Here's the drawing with two shaded views (mm, measured from the low corner). I have some questions. Coordinates: 2 decimals unless noted, no trailing zeros. Order: outer loops, then holes, each group sorted by start corner. A loop starts at its lowest first (then second) coordinate and runs counter-clockwise, first axis right, second up. Notation, with made-up numbers: (37, 85.5) - (76, 85.5) arc R22 cw to (76, 104.5) - close; hole circle Ø11 at (43.25, 25.5). An arc over 180 degrees is marked (long way). Answer as a JSON object with one key per item and string values. Group by question number.
(1) Please list where these lines run through material, in increasing order: probe 1 along Z at (x, y) = (7.5, 2.5); probe 2 along X at (y, z) = (15, 180); probe 3 along X at (y, z) = (11.25, 20).
(2) Imagine slicing it at D-D, the plane z = 145. Write out the boundary of the cut face in (x, y), and give its area (3 significant figures).
(3) Imagine slicing it at A-A, the plane z = 190. Write out the boundary of the cut face in (x, y).
(4) Imagine slicing it at B-B, the plane x = 100. Write out the boundary of the cut face in (y, z), and give its area (3 significant figures).
(5) Will these pins go through, and if not, where does the flat tip stop? P1, Ø9.5, axis at x = 42.5, z = 180, coming from the -Y side; P2, Ø5, axis at y = 10, z = 20, coming from the +X side.
(6) Imagine slicing it at C-C, the plane y = 4.75. Give the number of separate pieces and of enclosed holes in the cut face, and give its area (3 significant figures).
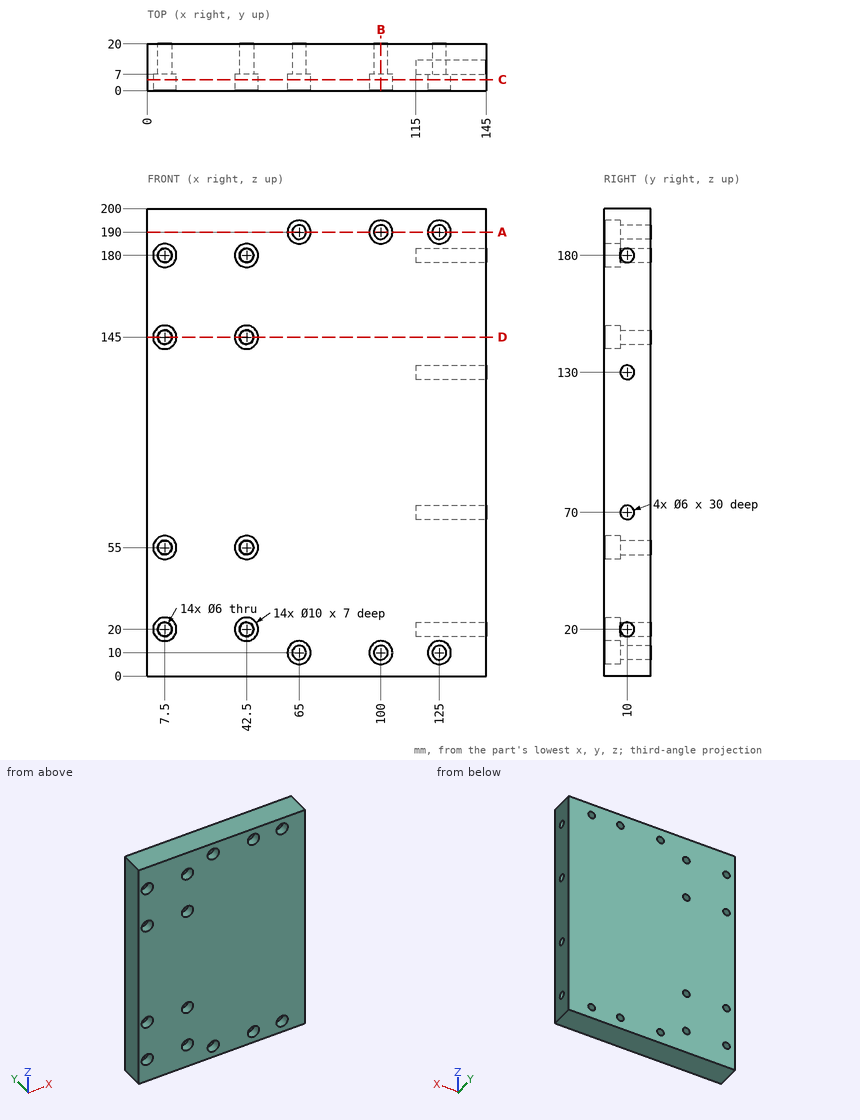
Result set:
{
 "1": {"probe 1": "z = 0 to 15, 25 to 50, 60 to 140, 150 to 175, 185 to 200", "probe 2": "x = 0 to 4.5, 10.5 to 39.5, 45.5 to 145", "probe 3": "x = 0 to 4.5, 10.5 to 39.5, 45.5 to 115"},
 "2": {"outline": "(0, 0) - (2.5, 0) - (2.5, 7) - (4.5, 7) - (4.5, 20) - (0, 20) - close; (10.5, 7) - (12.5, 7) - (12.5, 0) - (37.5, 0) - (37.5, 7) - (39.5, 7) - (39.5, 20) - (10.5, 20) - close; (45.5, 7) - (47.5, 7) - (47.5, 0) - (145, 0) - (145, 20) - (45.5, 20) - close", "area": "2,600 mm^2"},
 "3": {"outline": "(0, 0) - (60, 0) - (60, 7) - (62, 7) - (62, 20) - (0, 20) - close; (68, 7) - (70, 7) - (70, 0) - (95, 0) - (95, 7) - (97, 7) - (97, 20) - (68, 20) - close; (103, 7) - (105, 7) - (105, 0) - (120, 0) - (120, 7) - (122, 7) - (122, 20) - (103, 20) - close; (128, 7) - (130, 7) - (130, 0) - (145, 0) - (145, 20) - (128, 20) - close"},
 "4": {"outline": "(0, 0) - (20, 0) - (20, 7) - (7, 7) - (7, 5) - (0, 5) - close; (0, 15) - (7, 15) - (7, 13) - (20, 13) - (20, 187) - (7, 187) - (7, 185) - (0, 185) - close; (0, 195) - (7, 195) - (7, 193) - (20, 193) - (20, 200) - (0, 200) - close", "area": "3,700 mm^2"},
 "5": {"P1": "stops at y = 7", "P2": "stops at x = 115"},
 "6": {"separate pieces": "1", "enclosed holes": "14", "area": "27,900 mm^2"}
}
